Geometry: see drawing. Coordinates: mm, zero at the bounding-box minimum. A direction names the side the tool comes from. Round coordinates to 2 decimals unless told otherwise and drop trailing zeros. Write each loop counter-clockwise with the first axis right and the second up, starting at its lowest first coordinate (ties: lowest second). Pieces come first, ordered by that corner, then holes. Notation, with made-up numbers: (85, -30.5) - (112, -30.5) arc R21 ccw to (112, -10.5) - close; hole circle Ø3 at (2, 59). An arc over 180 degrees is marked (long way). Use a Markdown table: item, result. Add a question column.
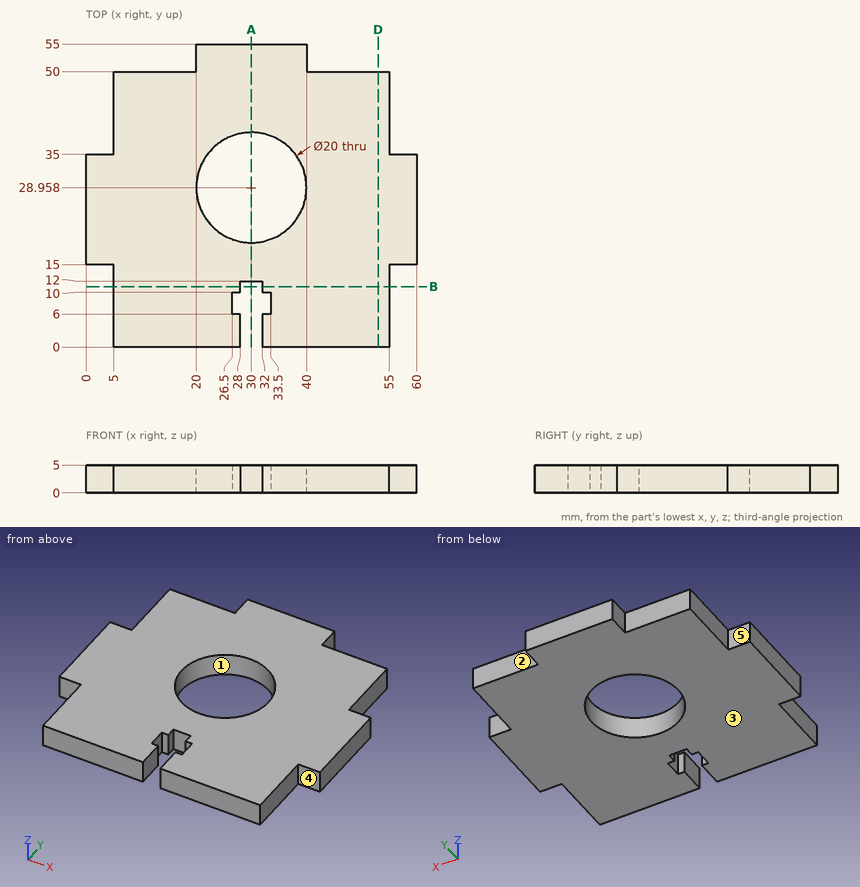
1) Set-up query: the marked faces 3, 4 and 5. Return all of +Z, -Z, +X, -X, +Y, -Y with unobstructed straight access to the full face (end or side cutting, diameter ignored); none if empty.
2) Section B-B, the plane y = 11. Return the cut outline in (x, z).
3) Section D-D, the plane x = 53. Return the cut outline in (y, z).
4) Pin query (flat end, axial travel): P1, Ø1.5, axis at x = 13.5, z = 3.5, coming from the +Y side; P2, Ø2.5, axis at x = 57, z = 1.5, coming from the +Y side; P3, Ø2, axis at x = 29.5, z = 3, coming from the -Y side. Return the tip coordinate at first contact, or that it passes through.
5) Draft query along X for the marked faces 1 and 2. Return one class per face: released by +X, released by -X, zero draft, split by the parting line, or undercut.
6) Material intervals for L1, parallel to X at y = 8, z = 1.75; L2, parallel to Y at x = 30, z = 1.3; L3, parallel to X at y = 5.5, z = 2.25, sorted ascending. Write a range as from..to.
7) Section A-A, the plane x = 30. Return the cut outline in (y, z).
Output values:
| question | item | result |
|---|---|---|
| 1 | face 3 | -Z, +X, -X, +Y, -Y |
| 1 | face 4 | +Z, -Z, +X, -Y |
| 1 | face 5 | +Z, -Z, -X, +Y |
| 2 | outline | (5, 0) - (28, 0) - (28, 5) - (5, 5) - close; (32, 0) - (55, 0) - (55, 5) - (32, 5) - close |
| 3 | outline | (0, 0) - (50, 0) - (50, 5) - (0, 5) - close |
| 4 | P1 | stops at y = 50 |
| 4 | P2 | stops at y = 35 |
| 4 | P3 | stops at y = 12 |
| 5 | face 1 | undercut |
| 5 | face 2 | zero draft |
| 6 | L1 | x = 5..26.5, 33.5..55 |
| 6 | L2 | y = 12..18.96, 38.96..55 |
| 6 | L3 | x = 5..28, 32..55 |
| 7 | outline | (12, 0) - (18.96, 0) - (18.96, 5) - (12, 5) - close; (38.96, 0) - (55, 0) - (55, 5) - (38.96, 5) - close |
